from build123d import *

# Parameters (mm, degrees)
SKETCH_1_R      = 1.65
EXTRUDE_1_DEPTH = 10


with BuildPart() as part:
    # 草图1 → 凸台-拉伸1 (new body)
    with BuildSketch(Plane(origin=(56.415924247, 0, 0), x_dir=(0, 0, -1), z_dir=(1, 0, 0))):
        with BuildLine():
            Line((-55.264392442, -53.153642626), (-87.583702197, -84.606168615))
            ThreePointArc((-87.583702197, -84.606168615), (-112.572118878, -90.553138734), (-88.412490375, -99.276657086))
            Line((-88.412490375, -99.276657086), (-46.780021188, -57.644187899))
            ThreePointArc((-46.780021188, -57.644187899), (-45.496623318, -55.576307852), (-45.264392442, -53.153642626))
            Line((-45.264392442, -53.153642626), (-45.264392442, -21.663090289))
            ThreePointArc((-45.264392442, -21.663090289), (-50.264392442, -16.663090289), (-55.264392442, -21.663090289))
            Line((-55.264392442, -21.663090289), (-55.264392442, -53.153642626))
        make_face()
        with Locations((-50.264392442, -21.663090289)):
            Circle(SKETCH_1_R, mode=Mode.SUBTRACT)
        with Locations((-99.19033753, -91.309123254)):
            Circle(SKETCH_1_R, mode=Mode.SUBTRACT)
    extrude(amount=EXTRUDE_1_DEPTH)


solid = part.part
Input: part model. Units: mm. Frame: model coordinates. A direction names the side the tool comes from. Round coordinates to 2 decimals unless told otherwise and drop trailing zeros. Write each loop counter-clockwise with the first axis right and the second up, starting at its lowest first coordinate (ties: lowest second). Pieces come first, ordered by that corner, then holes.
1) Cut plane B-B (y = -48). Return the cut outline in (x, z), then the cut area to 4 significant figures.
2) Contact query for flat-ended pins moving along their axis: P1, Ø3, axis at x = 61, y = -44, coming from the -Z side; P2, Ø3, axis at x = 63.5, z = 87.5, coming from the +Y side; P3, Ø1.5, axis at y = -48.5, z = 56.5, coming from the -X side; P4, Ø5, axis at x = 60, z = 89.5, coming from the +Y side. Output: stop coordinate, or through.
3) Reachability of faces 5 (the cylindrical face through (61.35, -92.92, 99.55)), 6 (the flat face through (61.35, -68.66, 71.2)) from +Z, -Z, +X, -X, +Y, -Y: full face, straight path, thin tool, end or side. Return the list, or none.
4) Draft query along Z for faces 1 (the flat face through (56.416, -74, 74)), 2 (the cylindrical face through (61.346, -23.274, 50.622)), 3 (the flat face through (61, -37, 55.264)), 4 (the cylindrical face through (61.346, -90.074, 112.536)). Return one class per face: pulls with the +Z half, pulls with the -Z half, needs draft (parallel to the pull), parting line crosses it, or undercut.
5) Cut plane A-A (x = 65.25). Return the cut outline in (y, z).
6) Cut plane C-C (z = 89.5). Return the cut outline in (x, y), then the cut area to 3 significant figures.
7) Ray query, L1, parallel to Z at x = 58.5, y = -44.5; L2, parallel to Y at x = 61, z = 100; L3, parallel to Y at x = 63.25, z = 49.5. Return the intervals inside material, ascending.
Geometry says:
1. outline: (56.42, 45.26) - (66.42, 45.26) - (66.42, 55.26) - (56.42, 55.26) - close
1. area: 100.0 mm2
2. P1: stops at z = 45.26
2. P2: stops at y = -82.6
2. P3: passes through
2. P4: stops at y = -80
3. face 5: +X, -X
3. face 6: +X, -X, +Y
4. face 1: needs draft
4. face 2: undercut
4. face 3: pulls with the +Z half
4. face 4: undercut
5. outline: (-99.28, 88.41) - (-57.64, 46.78) arc R5.34 ccw to (-53.15, 45.26) - (-21.66, 45.26) arc R5 ccw to (-21.66, 55.26) - (-53.15, 55.26) - (-84.61, 87.58) arc R13.4 ccw (long way) to start; hole circle Ø3.3 at (-91.31, 99.19); hole circle Ø3.3 at (-21.66, 50.26)
6. outline: (56.42, -100.57) - (66.42, -100.57) - (66.42, -82.05) - (56.42, -82.05) - close
6. area: 185 mm2
7. L1: z = 45.26 to 55.26
7. L2: y = -104.69 to -92.75, -89.87 to -77.93
7. L3: y = -60.36 to -23.13, -20.2 to -16.72
